```python
from build123d import *

# Parameters (mm, degrees)
SKETCH3_R           = 1.5
BOSS_EXTRUDE1_DEPTH = 3


with BuildPart() as part:
    # Sketch3 → Boss-Extrude1 (new body)
    with BuildSketch(Plane.XY):
        with BuildLine():
            Line((-9.681295011, -10.548579379), (-2.586204824, 1.520376469))
            ThreePointArc((-2.586204824, 1.520376469), (-1.520557397, 2.586098452), (-0.071160516, 2.999155911))
            Line((-0.071160516, 2.999155911), (94.857678968, 5.25151804))
            ThreePointArc((94.857678968, 5.25151804), (100.991739474, -0.432058845), (95.486888577, -6.727006113))
            Line((95.486888577, -6.727006113), (-6.851645898, -15.059062012))
            ThreePointArc((-6.851645898, -15.059062012), (-9.636397947, -13.663244049), (-9.681295011, -10.548579379))
        make_face()
        with Locations((-7.095090187, -12.068955847)):
            Circle(SKETCH3_R, mode=Mode.SUBTRACT)
        Circle(SKETCH3_R, mode=Mode.SUBTRACT)
    extrude(amount=BOSS_EXTRUDE1_DEPTH)


solid = part.part
```
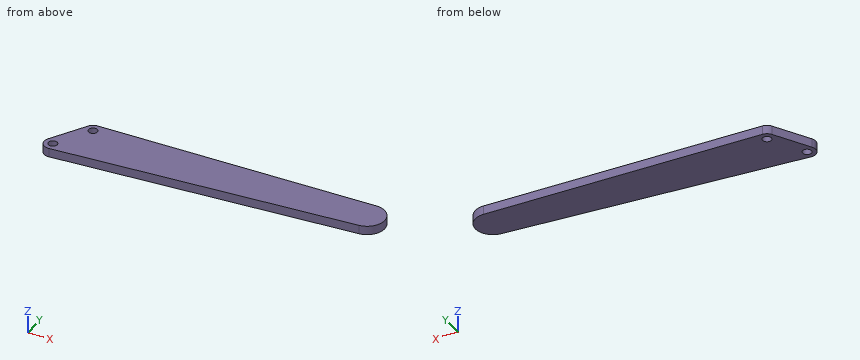
Here's how the part is built. I have some questions about the finished solid (model axes, mm). Round coordinates to 2 decimals unless told otherwise and drop trailing zeros. Write each loop counter-clockwise with the first axis right and the second up, starting at its lowest first coordinate (ties: lowest second). Pieces come first, ordered by that corner, then holes.
Q1. If we section it at D-D on x = 83.5: Write out the boundary of the cut face in (y, z), plus the area to 3 significant figures.
Q2. If we section it at A-A on y = 0: Write out the boundary of the cut face in (x, z), plus the area to 3 significant figures.
Q3. Please list where these lines run through material, in increasing order: probe 1 along X at (y, z) = (0.5, 0.4); probe 2 along Y at (x, z) = (0, 1.25); probe 3 along Y at (x, z) = (-1, 2.25).
Q4. If we section it at B-B on z = 1.1: Write out the boundary of the cut face in (x, y).
Q5. If we section it at C-C on x = 30.5: Write out the boundary of the cut face in (y, z), plus the area to 3 significant figures.
Answer below:
1. outline: (-7.7, 0) - (4.98, 0) - (4.98, 3) - (-7.7, 3) - close
1. area: 38.1 mm2
2. outline: (-3.48, 0) - (-1.5, 0) - (-1.5, 3) - (-3.48, 3) - close; (1.5, 0) - (100.95, 0) - (100.95, 3) - (1.5, 3) - close
2. area: 304 mm2
3. probe 1: x = -3.19 to -1.41, 1.41 to 100.87
3. probe 2: y = -14.5 to -1.5, 1.5 to 3
3. probe 3: y = -14.58 to -1.12, 1.12 to 2.83
4. outline: (-9.68, -10.55) arc R3 ccw to (-6.85, -15.06) - (95.49, -6.73) arc R6 ccw to (94.86, 5.25) - (-0.07, 3) arc R3 ccw to (-2.59, 1.52) - close; hole circle Ø3 at (-7.1, -12.07); hole circle Ø3 at (0, 0)
5. outline: (-12.02, 0) - (3.72, 0) - (3.72, 3) - (-12.02, 3) - close
5. area: 47.2 mm2
